Design review of the part built by this model. Coordinates are the model's own, in mm. A direction names the side the tool comes from. Coordinates: 2 decimals unless noted, no trailing zeros. Write each loop counter-clockwise with the first axis right and the second up, starting at its lowest first coordinate (ties: lowest second). Pieces come first, ordered by that corner, then holes. Notation, with made-up numbers: (-9.75, 38) - (21.25, 38) arc R15 ccw to (21.25, 44) - close; hole circle Ø5 at (89, 47). An arc over 180 degrees is marked (long way). One line per item, written item: value.
Autodesk Inventor part; units mm, degrees
ref_plane "Work Plane1" through (-38.5, 0, -61) normal (-1, 0, 0) x (0, 0, 1)
ref_plane "Work Plane2" through (0, 1.5, 0) normal (0, 1, 0) x (1, 0, 0)
ref_plane "YZ Plane" through (0, 0, 0) normal (1, 0, 0) x (0, 1, 0)
sketch "Sketch1" plane through (0, 0, 0) normal (0, 1, 0) x (-1, 0, 0)
  line L0 (38, 60.75) -> (-38, 60.75)
  line L1 (-38, 60.75) -> (-38, -60.75)
  line L2 (-38, -60.75) -> (38, -60.75)
  line L3 (38, -60.75) -> (38, 60.75)
  line L4 (0, 60.75) -> (0, -60.75) construction
  line L5 (-6.5, 39.25) -> (-25.5, 39.25)
  line L6 (-26.5, 38.25) -> (-26.5, 19.25)
  line L7 (-25.5, 18.25) -> (-6.5, 18.25)
  line L8 (-5.5, 19.25) -> (-5.5, 38.25)
  arc A0 (-5.5, 38.25) -> (-6.5, 39.25) centre (-6.5, 38.25) ccw
  arc A1 (-6.5, 18.25) -> (-5.5, 19.25) centre (-6.5, 19.25) ccw
  arc A2 (-26.5, 19.25) -> (-25.5, 18.25) centre (-25.5, 19.25) ccw
  arc A3 (-25.5, 39.25) -> (-26.5, 38.25) centre (-25.5, 38.25) ccw
  circle A4 centre (35.5, 57.65) radius 1
  circle A5 centre (-35.5, 57.65) radius 1
  line L9 (0, 0) -> (-51.842, 0) construction
  circle A6 centre (35.5, -57.75) radius 1
  circle A7 centre (-35.5, -57.75) radius 1
  line L10 (6.5, 39.25) -> (25.5, 39.25)
  line L11 (26.5, 38.25) -> (26.5, 19.25)
  line L12 (25.5, 18.25) -> (6.5, 18.25)
  line L13 (5.5, 19.25) -> (5.5, 38.25)
  arc A8 (6.5, 39.25) -> (5.5, 38.25) centre (6.5, 38.25) ccw
  arc A9 (5.5, 19.25) -> (6.5, 18.25) centre (6.5, 19.25) ccw
  arc A10 (25.5, 18.25) -> (26.5, 19.25) centre (25.5, 19.25) ccw
  arc A11 (26.5, 38.25) -> (25.5, 39.25) centre (25.5, 38.25) ccw
  line L14 (25.5, -9.75) -> (6.5, -9.75)
  arc A12 (25.5, -9.75) -> (26.5, -8.75) centre (25.5, -8.75) ccw
  arc A13 (5.5, -8.75) -> (6.5, -9.75) centre (6.5, -8.75) ccw
  arc A14 (-6.5, -9.75) -> (-5.5, -8.75) centre (-6.5, -8.75) ccw
  line L15 (-25.5, -9.75) -> (-6.5, -9.75)
  arc A15 (-26.5, -8.75) -> (-25.5, -9.75) centre (-25.5, -8.75) ccw
  line L16 (-6.5, 11.25) -> (-25.5, 11.25)
  line L17 (-26.5, 10.25) -> (-26.5, -8.75)
  line L18 (-5.5, -8.75) -> (-5.5, 10.25)
  arc A16 (-5.5, 10.25) -> (-6.5, 11.25) centre (-6.5, 10.25) ccw
  arc A17 (-25.5, 11.25) -> (-26.5, 10.25) centre (-25.5, 10.25) ccw
  line L19 (5.5, -8.75) -> (5.5, 10.25)
  line L20 (26.5, 10.25) -> (26.5, -8.75)
  arc A18 (6.5, 11.25) -> (5.5, 10.25) centre (6.5, 10.25) ccw
  line L21 (6.5, 11.25) -> (25.5, 11.25)
  arc A19 (26.5, 10.25) -> (25.5, 11.25) centre (25.5, 10.25) ccw
  point P0 (-26.5, 18.25)
  point P1 (-26.5, 39.25)
  point P2 (-5.5, 18.25)
  point P3 (26.5, 18.25)
  point P4 (26.5, 39.25)
  point P5 (5.5, 18.25)
  point P6 (26.5, -9.75)
  point P7 (5.5, -9.75)
  point P8 (-5.5, -9.75)
  point P9 (-26.5, -9.75)
  point P10 (-26.5, 11.25)
  point P11 (26.5, 11.25)
  dimension "d0" = 121.5
  dimension "d1" = 76
  dimension "d2" = 21
  dimension "d3" = 21
  dimension "d5" = 1
  dimension "d15" = 2
  dimension "d30" = 3.1
  dimension "d31" = 2.5
  dimension "d33" = 3
  dimension "d52" = 5.5
  dimension "d55" = 28
  dimension "d60" = 100
  dimension "d73" = 2.5
  dimension "d74" = 2.5
  dimension "d75" = 2.5
extrude "Extrusion6" add sketch "Sketch1" along normal blind 1.6
hole "Hole3" at (-35.5, 0, 57.65) at (35.5, 0, 57.65) at (-35.5, 0, -57.75) at (35.5, 0, -57.75) direction (0, 1, 0) diameter 2 depth 8 tip angle 118 countersink diameter 3 countersink angle 90
ref_plane "Work Plane1" through (-38.5, 0, -61) normal (-1, 0, 0) x (0, 0, 1)
sketch "Sketch2" plane through (-38.5, 0, -61) normal (-1, 0, 0) x (0, 0, 1)
  line L0 (0, 0) -> (121.75, 0)
  line L1 (121.75, 0) -> (121.75, 1.6)
  line L2 (121.75, 1.6) -> (125.924, 0)
  line L3 (121.75, 0) -> (125.924, 0)
  point P0 (61, 0)
  point P1 (121.924, 0)
ref_plane "Work Plane2" through (0, 1.5, 0) normal (0, 1, 0) x (1, 0, 0)
extrude "Extrusion8" add sketch "Sketch2" against normal up to surface (76.5 mm away)
sketch "Sketch4" plane through (0, 1.6, 0) normal (0, 1, 0) x (1, 0, 0)
  arc A0 (6.5, 9.75) -> (5.5, 8.75) centre (6.5, 8.75) ccw
  line L0 (6.5, 9.75) -> (25.5, 9.75)
  arc A1 (26.5, 8.75) -> (25.5, 9.75) centre (25.5, 8.75) ccw
  line L1 (26.5, 8.75) -> (26.5, -10.25)
  arc A2 (25.5, -11.25) -> (26.5, -10.25) centre (25.5, -10.25) ccw
  line L2 (25.5, -11.25) -> (6.5, -11.25)
  arc A3 (5.5, -10.25) -> (6.5, -11.25) centre (6.5, -10.25) ccw
  line L3 (5.5, -10.25) -> (5.5, 8.75)
  arc A4 (-5.5, 8.75) -> (-6.5, 9.75) centre (-6.5, 8.75) ccw
  line L4 (-5.5, 8.75) -> (-5.5, -10.25)
  arc A5 (-6.5, -11.25) -> (-5.5, -10.25) centre (-6.5, -10.25) ccw
  line L5 (-6.5, -11.25) -> (-25.5, -11.25)
  arc A6 (-26.5, -10.25) -> (-25.5, -11.25) centre (-25.5, -10.25) ccw
  line L6 (-26.5, -10.25) -> (-26.5, 8.75)
  arc A7 (-25.5, 9.75) -> (-26.5, 8.75) centre (-25.5, 8.75) ccw
  line L7 (-25.5, 9.75) -> (-6.5, 9.75)
  arc A8 (-5.5, -19.25) -> (-6.5, -18.25) centre (-6.5, -19.25) ccw
  line L8 (-5.5, -19.25) -> (-5.5, -38.25)
  arc A9 (-6.5, -39.25) -> (-5.5, -38.25) centre (-6.5, -38.25) ccw
  line L9 (-6.5, -39.25) -> (-25.5, -39.25)
  arc A10 (-26.5, -38.25) -> (-25.5, -39.25) centre (-25.5, -38.25) ccw
  line L10 (-26.5, -38.25) -> (-26.5, -19.25)
  arc A11 (-25.5, -18.25) -> (-26.5, -19.25) centre (-25.5, -19.25) ccw
  line L11 (-25.5, -18.25) -> (-6.5, -18.25)
  arc A12 (6.5, -18.25) -> (5.5, -19.25) centre (6.5, -19.25) ccw
  line L12 (6.5, -18.25) -> (25.5, -18.25)
  arc A13 (26.5, -19.25) -> (25.5, -18.25) centre (25.5, -19.25) ccw
  line L13 (26.5, -19.25) -> (26.5, -38.25)
  arc A14 (25.5, -39.25) -> (26.5, -38.25) centre (25.5, -38.25) ccw
  line L14 (25.5, -39.25) -> (6.5, -39.25)
  arc A15 (5.5, -38.25) -> (6.5, -39.25) centre (6.5, -38.25) ccw
  line L15 (5.5, -38.25) -> (5.5, -19.25)
  circle A16 centre (35.5, 57.75) radius 1
  circle A17 centre (-35.5, 57.75) radius 1
  circle A18 centre (35.5, -57.65) radius 1
  circle A19 centre (-35.5, -57.65) radius 1
  line L16 (-38, -60.75) -> (38, -60.75)
  line L17 (38, -60.75) -> (38, 60.75)
  line L18 (38, 60.75) -> (-38, 60.75)
  line L19 (-38, 60.75) -> (-38, -60.75)
  line L20 (6.5, -40.45) -> (25.5, -40.45)
  arc A20 (25.5, -40.45) -> (27.7, -38.25) centre (25.5, -38.25) ccw
  line L21 (27.7, -38.25) -> (27.7, -19.25)
  arc A21 (27.7, -19.25) -> (25.5, -17.05) centre (25.5, -19.25) ccw
  line L22 (25.5, -17.05) -> (6.5, -17.05)
  arc A22 (6.5, -17.05) -> (4.3, -19.25) centre (6.5, -19.25) ccw
  line L23 (4.3, -19.25) -> (4.3, -38.25)
  arc A23 (4.3, -38.25) -> (6.5, -40.45) centre (6.5, -38.25) ccw
  line L24 (6.5, -12.45) -> (25.5, -12.45)
  arc A24 (25.5, -12.45) -> (27.7, -10.25) centre (25.5, -10.25) ccw
  line L25 (27.7, -10.25) -> (27.7, 8.75)
  arc A25 (27.7, 8.75) -> (25.5, 10.95) centre (25.5, 8.75) ccw
  line L26 (25.5, 10.95) -> (6.5, 10.95)
  arc A26 (6.5, 10.95) -> (4.3, 8.75) centre (6.5, 8.75) ccw
  line L27 (4.3, 8.75) -> (4.3, -10.25)
  arc A27 (4.3, -10.25) -> (6.5, -12.45) centre (6.5, -10.25) ccw
  point P0 (0, 0)
  dimension "d69" = 1.2
  dimension "d70" = 1.2
extrude "Extrusion9" add sketch "Sketch4" along normal blind 1.6 contours A23 L23 A22 L22 A21 L21 A20 L20 | A27 L27 A26 L26 A25 L25 A24 L24
mirror "Mirror1" about plane through (0, 0, 0) normal (1, 0, 0) of "Extrusion9"
equation "\"d73\" = d31"
properties part number "front_cover" material "Aluminum 6061"
1. Consider section B-B, the plane z = 8.5. Write out the cut boundary in (x, y).
Answer block:
outline: (-38, 0) - (-26.5, 0) - (-26.5, 3.2) - (-27.7, 3.2) - (-27.7, 1.6) - (-38, 1.6) - close; (-5.5, 0) - (5.5, 0) - (5.5, 3.2) - (4.3, 3.2) - (4.3, 1.6) - (-4.3, 1.6) - (-4.3, 3.2) - (-5.5, 3.2) - close; (26.5, 0) - (38, 0) - (38, 1.6) - (27.7, 1.6) - (27.7, 3.2) - (26.5, 3.2) - close
2. For faces 3 (the face through (15, 3.2, 12)), 4 (the face through (-16, 2, 18.25)), list the 3-axis set-ups (+Z, -Z, +X, -X, +Y, -Y) from which the entire face can be reached by the end or side of a thin tool; tool diameter is ignored.
Answer block:
face 3: +Z, -Z, +X, -X, +Y
face 4: +Y, -Y
3. Wall thickness on line 1 along X through (y, z) = (1.15, -57.75); line 2 along Z through (x, y) = (-7, 2.7); line 3 along X through (y, z) = (2.2, 20.5): over which ranges is each line inside the solid? List them lowest first.
Answer block:
line 1: x = -38 to -36.5, -34.5 to 34.5, 36.5 to 38
line 2: z = -10.95 to -9.75, 11.25 to 12.45, 17.05 to 18.25, 39.25 to 40.45
line 3: x = -27.7 to -26.5, -5.5 to -4.3, 4.3 to 5.5, 26.5 to 27.7
4. Insertion check: pin 1 Ø1.3 at (y, z) = (2, -2.5) entering from -X; pin 2 Ø0.8 at (y, z) = (2.5, 32) entering from -X; pin 3 Ø0.5 at (x, y) = (18.5, 2.5) entering from +Z. Each pin has a flat end and moves straight along its axis. Give the tip position at first contact, or say it passes through.
Answer block:
pin 1: stops at x = -38
pin 2: stops at x = -27.7
pin 3: stops at z = 40.45
5. Consider section D-D, the plane z = 44. Write out the cut boundary in (x, y).
Answer block:
outline: (-38, 0) - (38, 0) - (38, 1.6) - (-38, 1.6) - close
6. Mouldability with a two-part tool opening along X and no side actions: class faces 1 (the face through (-1, 0, 1)), 2 (the face through (26.5, 2, 29)) as released by +X, released by -X, zero draft, split by the parting line, or undercut.
Answer block:
face 1: zero draft
face 2: undercut
7. Consider section A-A, the plane x = -22.5. Write out the cut boundary in (y, z), then the cut area to 3 significant figures.
Answer block:
outline: (0, -60.75) - (1.6, -60.75) - (1.6, -10.95) - (3.2, -10.95) - (3.2, -9.75) - (0, -9.75) - close; (0, 11.25) - (3.2, 11.25) - (3.2, 12.45) - (1.6, 12.45) - (1.6, 17.05) - (3.2, 17.05) - (3.2, 18.25) - (0, 18.25) - close; (0, 39.25) - (3.2, 39.25) - (3.2, 40.45) - (1.6, 40.45) - (1.6, 60.75) - (0, 64.92) - close
area: 138 mm^2
8. Consider section C-C, the plane y = 2.1. Give the number of separate pieces and of enclosed holes in the cut face, then the cut area to 3 significant figures.
Answer block:
separate pieces: 4
enclosed holes: 4
area: 413 mm^2
